Verification items for the finished model (mm, model axes). A direction names the side the tool comes from. Coordinates: 2 decimals unless noted, no trailing zeros. Order: outer loops, then holes, each group sorted by start corner. A loop starts at its lowest first (then second) coordinate and runs counter-clockwise, first axis right, second up. Notation, with made-up numbers: (73.5, 63) -> (95.5, 63) arc R9 cw to (95.5, 68) -> close; hole circle Ø7 at (-23.5, 78.5). An arc over 180 degrees is marked (long way). Use CSV: the item, a comma, the result in double quotes. Start each with the question number.
1) Release check for a two-part mould opening along X. For faces 3 (the flat face through (0, -5, 113)), 4 (the flat face through (4, 0, 113)), 5 (the flat face through (0, 4, 113)), 6 (the flat face through (5, 0, 113)) record: released by +X, released by -X, zero draft, split by the parting line, or undercut.
2) Sectioned sample at B-B on z = 101.5. Record the boundary of the cut face in (x, y), then the cut area to 3 significant figures.
3) Sectioned sample at C-C on y = 0. Give the number of separate pieces and of enclosed holes in the cut face, then the cut area to 3 significant figures.
4) Sectioned sample at A-A on x = 0. Record the boundary of the cut face in (y, z), then the cut area to 3 significant figures.
5) Scan lines: line 1 along Z through (x, y) = (0, -4.6); line 2 along Y through (x, z) = (3.5, 93.5). Record each from-to range of solid material in increasing order.
6) Tool access check on faces 1 (the flat face through (-4.5, 0.1, 0)), 2 (the flat face through (0, -4, 113)). Record the directions out of +Z, -Z, +X, -X, +Y, -Y that give a thin tool (end or side, any length) a straight path to the whole face; none if there is none.
from build123d import *

# Parameters (mm, degrees)
F0_W     = 10
F0_H     = 10
F0_W_2   = 8
F0_H_2   = 8
F1_DEPTH = 230
F2_R     = 1.5
F3_DEPTH = 25
F4_R     = 1.5
F5_DEPTH = 25


with BuildPart() as f1:
    # F0 (on Top) → F1 (new body)
    with BuildSketch(Plane.XY):
        Rectangle(F0_W, F0_H)
        Rectangle(F0_W_2, F0_H_2, mode=Mode.SUBTRACT)
    extrude(amount=F1_DEPTH)

    # F2 (on face) → F3 (cut)
    with BuildSketch(Plane.YZ.offset(5)):
        with Locations((0, 80.5)):
            Circle(F2_R)
        with Locations((0, 15)):
            Circle(F2_R)
        with Locations((0, 149.5)):
            Circle(F2_R)
        with Locations((0, 215)):
            Circle(F2_R)
    extrude(amount=-F3_DEPTH, mode=Mode.SUBTRACT)

    # F4 (on face) → F5 (cut)
    with BuildSketch(Plane.XZ.offset(5)):
        with Locations((0, 5)):
            Circle(F4_R)
        with Locations((0, 225)):
            Circle(F4_R)
    extrude(amount=-F5_DEPTH, mode=Mode.SUBTRACT)


solid = f1.part
Answers follow:
1,face 3,"zero draft"
1,face 4,"undercut"
1,face 5,"undercut"
1,face 6,"released by +X"
2,outline,"(-5, -5) -> (5, -5) -> (5, 5) -> (-5, 5) -> close; hole (-4, -4) -> (4, -4) -> (4, 4) -> (-4, 4) -> close"
2,area,"36.0 mm²"
3,separate pieces,"10"
3,enclosed holes,"0"
3,area,"436 mm²"
4,outline,"(-5, 0) -> (-4, 0) -> (-4, 3.5) -> (-5, 3.5) -> close; (-5, 6.5) -> (-4, 6.5) -> (-4, 223.5) -> (-5, 223.5) -> close; (-5, 226.5) -> (-4, 226.5) -> (-4, 230) -> (-5, 230) -> close; (4, 0) -> (5, 0) -> (5, 3.5) -> (4, 3.5) -> close; (4, 6.5) -> (5, 6.5) -> (5, 223.5) -> (4, 223.5) -> close; (4, 226.5) -> (5, 226.5) -> (5, 230) -> (4, 230) -> close"
4,area,"448 mm²"
5,line 1,"z = 0 to 3.5, 6.5 to 223.5, 226.5 to 230"
5,line 2,"y = -5 to -4, 4 to 5"
6,face 1,"-Z, +X, -X, +Y, -Y"
6,face 2,"+Z, -Z"
